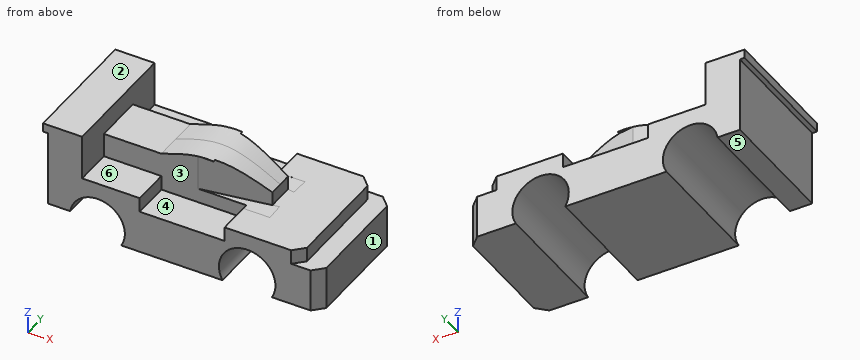
from build123d import *

# Parameters (mm, degrees)
F1_DEPTH = 31.75
F2_DEPTH = 12.7
F3_DEPTH = 12.7
F0_W     = 2.4479581043
F0_H     = 4.5006387227
F4_DEPTH = 31.75
F5_SIZE  = 5.08
F7_DEPTH = 17.78


with BuildPart() as f1:
    # F0 (on Front) → F1 (new body, symmetric)
    with BuildSketch(Plane.XZ):
        with BuildLine():
            Line((-37.2165674344, 5.0159874372), (-54.7461742535, 5.0159874372))
            Line((-54.7461742535, 5.0159874372), (-54.7461742535, 0.5153487145))
            Line((-54.7461742535, 0.5153487145), (-54.7461742535, -37.9826184362))
            Line((-54.7461742535, -37.9826184362), (-43.3364818902, -37.9826184362))
            ThreePointArc((-43.3364818902, -37.9826184362), (-28.3889674357, -26.1480412328), (-15.4376497281, -40.1390660554))
            ThreePointArc((-15.4376497281, -40.1390660554), (-15.9095240894, -43.7474911576), (-17.2934120834, -47.1132379025))
            Line((-17.2934120834, -47.1132379025), (34.3146193156, -47.1132379025))
            ThreePointArc((34.3146193156, -47.1132379025), (43.3213433173, -26.1879454869), (61.3312065818, -40.1390660554))
            ThreePointArc((61.3312065818, -40.1390660554), (60.8738629577, -43.7404651272), (59.5308654627, -47.1132379025))
            Line((59.5308654627, -47.1132379025), (84.3179924414, -47.0838975161))
            Line((84.3179924414, -47.0838975161), (84.3179924414, -25.180962868))
            Line((84.3179924414, -25.180962868), (74.4349635206, -25.180962868))
            Line((74.4349635206, -25.180962868), (74.4349635206, -17.7660211921))
            Line((74.4349635206, -17.7660211921), (45.3435182571, -17.7660211921))
            Line((45.3435182571, -17.7660211921), (35.4370600544, -17.7660211921))
            Line((35.4370600544, -17.7660211921), (35.4370600544, -25.180962868))
            Line((35.4370600544, -25.180962868), (-7.8752368445, -25.180962868))
            Line((-7.8752368445, -25.180962868), (-7.8752368445, -17.7660211921))
            Line((-7.8752368445, -17.7660211921), (-37.2165674344, -17.7660211921))
            Line((-37.2165674344, -17.7660211921), (-37.2165674344, -5.5272214778))
            Line((-37.2165674344, -5.5272214778), (-37.2165674344, 5.0159874372))
        make_face()
    extrude(amount=F1_DEPTH, both=True)

    # F0 (on Front) → F2 (join, symmetric)
    with BuildSketch(Plane.XZ):
        with BuildLine():
            add(Edge.make_bspline(
                [(-7.8752368445, -5.5272214778), (0.0340392295, -2.6463832002), (18.3779976424, 4.9271584445), (39.107106626, -7.3388037272), (45.3435182571, -10.7714328915)],
                knots=[0, 0, 0, 0, 0.4928089492, 1, 1, 1, 1], degree=3))
            Line((-7.8752368445, -5.5272214778), (-7.8752368445, -14.7637212649))
            Line((-7.8752368445, -14.7637212649), (-7.8752368445, -17.7660211921))
            Line((-7.8752368445, -17.7660211921), (-7.8752368445, -25.180962868))
            Line((-7.8752368445, -25.180962868), (35.4370600544, -25.180962868))
            Line((35.4370600544, -25.180962868), (35.4370600544, -17.7660211921))
            Line((35.4370600544, -17.7660211921), (45.3435182571, -17.7660211921))
            Line((45.3435182571, -17.7660211921), (45.3435182571, -10.7714328915))
        make_face()
    extrude(amount=F2_DEPTH, both=True)

    # F0 (on Front) → F3 (join, symmetric)
    with BuildSketch(Plane.XZ):
        Polygon((-7.8752368445, -5.5272214778), (-37.2165674344, -5.5272214778), (-37.2165674344, -17.7660211921), (-7.8752368445, -17.7660211921), (-7.8752368445, -14.7637212649), align=None)
    extrude(amount=F3_DEPTH, both=True)

    # F0 (on Front) → F4 (join, symmetric)
    with BuildSketch(Plane.XZ):
        with Locations((-55.9701533057, 2.7656680759)):
            Rectangle(F0_W, F0_H)
    extrude(amount=F4_DEPTH, both=True)

    # F5
    f5_edges = [f1.edges().sort_by_distance(p)[0] for p in [
        (74.434964, -31.75, -21.473492),
        (74.434964, 31.75, -21.473492),
        (84.317992, 31.75, -36.13243),
        (84.317992, -31.75, -36.13243),
    ]]
    chamfer(f5_edges, length=F5_SIZE)

    # F6 (on Top) → F7 (cut)
    with BuildSketch(Plane.XY):
        Polygon((7.4531887515, -13.2663722182), (7.5393404698, -15.4116023798), (49.021124661, -15.384102137), (48.6561246216, -6.2953792512), align=None)
        Polygon((48.6561246216, 6.2953792512), (49.021124661, 15.384102137), (7.5393404698, 15.4116023798), (7.4531887515, 13.2663722182), align=None)
    extrude(amount=-F7_DEPTH, mode=Mode.SUBTRACT)


solid = f1.part
Read the model definition and answer for the solid it produces. Units are mm, in the model's axes. Face numbers are marked on the shaded views. A direction names the side the tool comes from. Give positions to 0.01 mm unless a question says otherwise; leave off trailing zeros. Loops run counter-clockwise (first coordinate to the right, second up) from the corner with the lowest first, then second, coordinate; pieces in that order, holes last. Notation, with made-up numbers: (24.5, 83.25) - (36.5, 83.25) arc R14 cw to (36.5, 95.25) - close; hole circle Ø11 at (51.25, 83.5). An arc over 180 degrees is marked (long way). Answer as CSV lines item,"result". Start each with the question number.
1) Find section A-A (z = -14.5). Write down the section's boundary in (x, y).
2) Each of these flat-tipped pins is pushed along its axis until it touches: pin 1 Ø5 at (x, y) = (-11, 18) entering from +Z; pin 2 Ø19 at (y, z) = (4.5, -10.5) entering from -X; pin 3 Ø15 at (x, y) = (14, 25.5) entering from +Z; pin 4 Ø22.5 at (x, z) = (-29.47, -40.14) entering from +Y. Where does it stop, or does it pass through?
3) Find section B-B (y = -18). Write down the section's boundary in (x, z), then the cut area to 3 significant figures.
4) Find section C-C (x = -23). Write down the section's boundary in (y, z), then the cut area to 3 significant figures.
5) Which of the six approach directions +Z, -Z, +X, -X, +Y, -Y give full straight-line access (tool end or side, diameter ignored) to the marked faces 4, 5 and 6?
6) Determine the mould class of the marked faces 1, 2 and 3 for opening direction X: released by +X, released by -X, zero draft, split by the parting line, or undercut.
7) Find section D-D (z = -30). Write down the section's boundary in (x, y), then the cut area to 3 significant figures.
8) Straight lines are drawn through the part: L1, parallel to X at y = -22, z = -24.5; L2, parallel to X at y = 22, z = -41; L3, parallel to Z at x = 77, y = -12.5. For each, find the intervals that lie inside material, in ascending order. Write a range as from..to.
Findings below:
1,outline,"(-54.75, -31.75) - (-37.22, -31.75) - (-37.22, -12.7) - (10.8, -12.7) - (45.34, -6.86) - (45.34, 6.86) - (10.8, 12.7) - (-37.22, 12.7) - (-37.22, 31.75) - (-54.75, 31.75) - close"
2,pin 1,"z = -17.77"
2,pin 2,"x = -54.75"
2,pin 3,"z = -25.18"
2,pin 4,"through"
3,outline,"(-57.19, 0.52) - (-54.75, 0.52) - (-54.75, -37.98) - (-43.34, -37.98) arc R14.03 cw (long way) to (-17.29, -47.11) - (34.31, -47.11) arc R14.41 cw (long way) to (59.53, -47.11) - (84.32, -47.08) - (84.32, -25.18) - (74.43, -25.18) - (74.43, -17.77) - (35.44, -17.77) - (35.44, -25.18) - (-7.88, -25.18) - (-7.88, -17.77) - (-37.22, -17.77) - (-37.22, 5.02) - (-57.19, 5.02) - close"
3,area,"2,970 mm^2"
4,outline,"(-31.75, -27.69) - (31.75, -27.69) - (31.75, -17.77) - (12.7, -17.77) - (12.7, -5.53) - (-12.7, -5.53) - (-12.7, -17.77) - (-31.75, -17.77) - close"
4,area,"941 mm^2"
5,face 4,"+Z, -Y"
5,face 5,"-Z, -X, +Y, -Y"
5,face 6,"+Z, +X, -Y"
6,face 1,"released by +X"
6,face 2,"zero draft"
6,face 3,"undercut"
7,outline,"(-54.75, -31.75) - (-39.17, -31.75) - (-39.17, 31.75) - (-54.75, 31.75) - close; (-19.77, -31.75) - (36.69, -31.75) - (36.69, 31.75) - (-19.77, 31.75) - close; (57.16, -31.75) - (79.24, -31.75) - (84.32, -26.67) - (84.32, 26.67) - (79.24, 31.75) - (57.16, 31.75) - close"
7,area,"6,270 mm^2"
8,L1,"-54.75..-7.88, 35.44..74.43"
8,L2,"-15.46..32.54, 61.31..84.32"
8,L3,"-47.09..-25.18"
